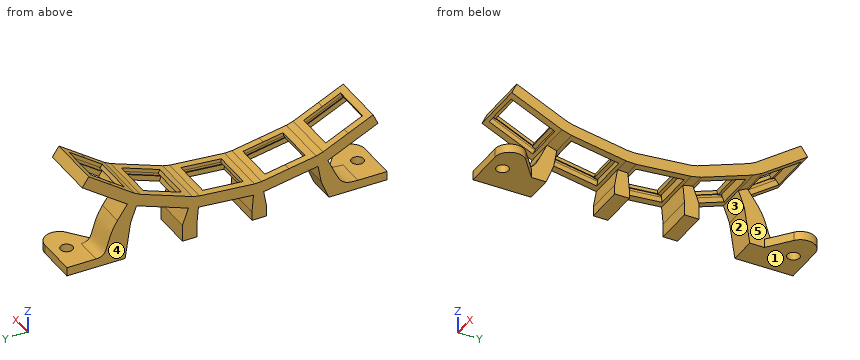
from build123d import *

# Parameters (mm, degrees)
PAD012_DEPTH      = 9.5
POCKET006_DEPTH   = 7
POCKET007_DEPTH   = 7.3
PAD013_DEPTH      = 4.1
PAD013_DEPTH_BACK = 9.5
PAD014_DEPTH      = 9.5
SKETCH025_R       = 2.1
PAD015_DEPTH      = 3


with BuildPart() as part:
    # Sketch020 → Pad012 (new body, symmetric)
    with BuildSketch(Plane.YZ):
        Polygon((-50.2140974459, 25.1635701277), (-41.604173469, 21.1486966411), (-32.9942494922, 17.1338231546), (-30.6406576873, 16.391738509), (-21.2849840337, 14.7420808212), (-11.9293103801, 13.0924231333), (-9.4638496319, 12.9847787924), (0, 13.8127583485), (9.4638496319, 14.6407379046), (11.8731622478, 15.1748696522), (20.8002421453, 18.4240610138), (29.7273220428, 21.6732523754), (31.9162958532, 22.8127600156), (39.698240274, 28.2617361609), (47.4801846947, 33.7107123063), (49.7744904401, 30.4341041291), (34.2106015986, 19.5361518385), (31.0954026161, 17.9144818922), (13.2412428211, 11.416099169), (9.8124726029, 10.6559591122), (-9.1152266609, 9), (-12.6239030908, 9.1531921213), (-31.335250398, 12.452507497), (-34.6847225392, 13.5085920065), (-51.9045704929, 21.5383389795), align=None)
    extrude(amount=PAD012_DEPTH, both=True)

    # Sketch021 → Pocket006 (cut, symmetric)
    with BuildSketch(Plane.YZ):
        Polygon((-47.9483279783, 24.1070244733), (-41.604173469, 21.1486966411), (-35.2600189598, 18.190368809), (-35.8516845262, 16.9215379071), (-34.6734844031, 16.3721341668), (-35.7722918836, 14.0157339205), (-43.294646516, 17.523465493), (-50.8170011484, 21.0311970654), (-49.7181936679, 23.3875973117), (-48.5399935447, 22.8381935715), align=None)
        Polygon((-30.1534810944, 12.2441296838), (-29.7019958324, 14.8046298416), (-28.4217457535, 14.5788872106), (-28.1786383048, 15.9576180648), (-21.2849840337, 14.7420808212), (-14.3913297626, 13.5265435775), (-14.6344372114, 12.1478127233), (-13.3541871324, 11.9220700923), (-13.8056723944, 9.3615699345), (-21.9795767444, 10.8028498091), align=None)
        Polygon((-8.1463979543, 11.6946931063), (-6.8513448468, 11.8079955719), (-6.9733628866, 13.2026681492), (0, 13.8127583485), (6.9733628866, 14.4228485477), (7.0953809265, 13.0281759704), (8.390434034, 13.1414784359), (8.6170389652, 10.5513722209), (0.348622971, 9.8279795561), (-7.9197930232, 9.1045868913), align=None)
        Polygon((14.2223937998, 16.0299200105), (20.8002421453, 18.4240610138), (27.3780904908, 20.818202017), (27.8569186914, 19.5026323479), (29.0785190985, 19.9472585343), (29.9677714711, 17.5040577202), (22.1683227186, 14.6652905306), (14.3688739661, 11.826523341), (13.4796215934, 14.2697241551), (14.7012220004, 14.7143503414), align=None)
        Polygon((33.7022853173, 22.3542388772), (34.7671829748, 23.0998882445), (33.964175964, 24.2467011065), (39.698240274, 28.2617361609), (45.432304584, 32.2767712154), (46.2353115949, 31.1299583534), (47.3002092525, 31.8756077207), (48.791507987, 29.7458124055), (41.9925460194, 24.9851279838), (35.1935840518, 20.2244435621), align=None)
    extrude(amount=POCKET006_DEPTH, both=True, mode=Mode.SUBTRACT)

    # Sketch022 → Pocket007 (cut, symmetric)
    with BuildSketch(Plane.YZ):
        Polygon((-48.4554698924, 23.0194551289), (-35.7671608739, 17.1027994645), (-35.8516845262, 16.9215379071), (-34.6734844031, 16.3721341668), (-35.0115790125, 15.6470879372), (-50.0562882773, 22.6625510822), (-49.7181936678, 23.3875973117), (-48.5399935447, 22.8381935715), align=None)
        Polygon((-28.387016118, 14.7758487612), (-14.5997075758, 12.3447742739), (-14.6344372114, 12.1478127233), (-13.3541871325, 11.9220700923), (-13.4931056746, 11.1342238899), (-29.8409143746, 14.0167836392), (-29.7019958324, 14.8046298416), (-28.4217457535, 14.5788872107), align=None)
        Polygon((-6.8687759954, 12.0072345116), (7.077949778, 13.2274149099), (7.0953809265, 13.0281759703), (8.390434034, 13.1414784359), (8.4601586282, 12.3445226773), (-8.0766733601, 10.8977373481), (-8.1463979543, 11.6946931063), (-6.8513448468, 11.8079955719), align=None)
        Polygon((14.6328179716, 14.9022888661), (27.788514663, 19.6905708716), (27.8569186915, 19.5026323479), (29.0785190985, 19.9472585342), (29.3521352133, 19.1955044372), (13.7532377079, 13.5179700589), (13.4796215934, 14.269724155), (14.7012220005, 14.7143503413), align=None)
        Polygon((34.6524676876, 23.2637186533), (46.1205963076, 31.2937887623), (46.2353115949, 31.1299583534), (47.3002092525, 31.8756077206), (47.7590704015, 31.2202860852), (34.1611464664, 21.6989172418), (33.7022853173, 22.3542388772), (34.7671829749, 23.0998882444), align=None)
    extrude(amount=POCKET007_DEPTH, both=True, mode=Mode.SUBTRACT)

    # Sketch023 → Pad013 (join, two sides)
    with BuildSketch(Plane.YZ) as pad013_sk:
        Polygon((-11.9293103801, 13.0924231333), (-9.4638496319, 12.9847787924), (-9.1152266609, 9), (-8.5922922044, 3.0228318114), (-8.5922922044, 0), (-13.6657921568, 0), (-13.6657921568, 3.2443456032), (-12.6239030908, 9.1531921213), align=None)
        Polygon((9.8124726029, 10.6559591122), (9.4638496319, 14.6407379046), (11.8731622478, 15.1748696522), (13.2412428211, 11.416099169), (15.2933636811, 5.7779434443), (15.2933636811, 0), (10.3354070593, 0), (10.3354070593, 4.6787909237), align=None)
    extrude(amount=PAD013_DEPTH)
    extrude(pad013_sk.sketch, amount=-PAD013_DEPTH_BACK)

    # Sketch024 → Pad014 (join)
    with BuildSketch(Plane.YZ):
        with BuildLine():
            Line((-45, 0), (-35, 0))
            Line((-35, 0), (-32.377139464, 6.5436609789))
            Line((-32.377139464, 6.5436609789), (-31.335250398, 12.452507497))
            Line((-31.335250398, 12.452507497), (-30.6406576873, 16.391738509))
            Line((-30.6406576873, 16.391738509), (-32.9942494922, 17.1338231546))
            Line((-32.9942494922, 17.1338231546), (-34.6847225392, 13.5085920065))
            Line((-34.6847225392, 13.5085920065), (-37.2204321096, 8.0707452842))
            add(Edge.make_bspline(
                [(-37.2204321096, 8.0707452842), (-39.0096732627, 4.233705249), (-40, 3), (-45, 3)],
                knots=[0, 0, 0, 0, 1, 1, 1, 1], degree=3))
            Line((-45, 3), (-45, 0))
        make_face()
        with BuildLine():
            Line((45, 3), (45, 0))
            Line((45, 0), (35, 0))
            Line((35, 0), (33.147523476, 12.2763261675))
            Line((33.147523476, 12.2763261675), (31.0954026161, 17.9144818922))
            Line((31.0954026161, 17.9144818922), (29.7273220428, 21.6732523754))
            Line((29.7273220428, 21.6732523754), (31.9162958532, 22.8127600156))
            Line((31.9162958532, 22.8127600156), (34.2106015986, 19.5361518385))
            Line((34.2106015986, 19.5361518385), (37.6520602167, 14.6212395727))
            add(Edge.make_bspline(
                [(37.6520602167, 14.6212395727), (42.2621193459, 8.0373928164), (40, 3), (45, 3)],
                knots=[0, 0, 0, 0, 1, 1, 1, 1], degree=3))
        make_face()
    extrude(amount=-PAD014_DEPTH)

    # Sketch025 → Pad015 (join)
    with BuildSketch(Plane.XY):
        with BuildLine():
            Line((0, 45), (-9.5, 45))
            Line((-9.5, 45), (-9.5, 55))
            Line((-9.5, 55), (4.5, 55))
            ThreePointArc((7.6224992299, 46.0948753465), (9.218348401, 51.6544450327), (4.5, 55))
            Line((7.6224992299, 46.0948753465), (0, 40))
            Line((0, 45), (0, 40))
        make_face()
        with Locations((0, 50)):
            Circle(SKETCH025_R, mode=Mode.SUBTRACT)
        with BuildLine():
            Line((0, -45), (-9.5, -45))
            Line((-9.5, -45), (-9.5, -55))
            Line((-9.5, -55), (4.5, -55))
            ThreePointArc((4.5, -55), (9.218348401, -51.6544450327), (7.6224992299, -46.0948753465))
            Line((7.6224992299, -46.0948753465), (0, -40))
            Line((0, -40), (0, -45))
        make_face()
        with Locations((0, -50)):
            Circle(SKETCH025_R, mode=Mode.SUBTRACT)
    extrude(amount=PAD015_DEPTH)


with BuildPart() as part_1:
    # Body003 placement: moved
    add(part.part.moved(Location((70, 5, 0))))


solid = part_1.part
Design review of the part built by this model. Coordinates are the model's own, in mm. Face numbers are marked on the shaded views. A direction names the side the tool comes from. Give positions to 0.01 mm unless a question says otherwise; leave off trailing zeros. Write each loop counter-clockwise with the first axis right and the second up, starting at its lowest first coordinate (ties: lowest second). Pieces come first, ordered by that corner, then holes. Notation, with made-up numbers: M -1,43.25 L 22,43.25 A30 ccw 22,76.25 Z; hole C -17,33 d3. An arc over 180 degrees is marked long. Answer as a JSON object with one key per item and string values. Group by question number.
1) For line 1 along X through (y, z) = (-32, 15.5); line 2 along X through (y, z) = (-5.5, 5); line 3 along Y through (x, z) = (66.5, 23), list the stretches that pass through material, from the lowest coordinate up.
2) We need section B-B (x = 64.5). Count the separate pieces of the cut face and the enclosed holes in it, and give its area (3 significant figures).
3) Mouldability with a two-part tool opening along X and no side actions: class the marked faces 3, 4 and 5 as released by +X, released by -X, zero draft, split by the parting line, or undercut.
4) We need section A-A (y = 24). Give the boundary of the cut face in (x, z), and give its area (3 significant figures).
5) Tool access review of the marked faces 1 and 2: name each direction out of +Z, -Z, +X, -X, +Y, -Y from which nothing blocks a thin tool from reaching the whole face with its end or side.
6) Clearance check with flat-ended pins moving along their axes: pin 1 Ø1.5 at (x, z) = (73, 15) entering from +Y; pin 2 Ø10 at (x, y) = (63, 29) entering from +Z; pin 3 Ø2 at (x, z) = (68, 4.5) entering from +Y; pin 4 Ø8 at (y, z) = (49, 26) entering from -X. State where each tip first meets the part, or that it passes through.
Answer key:
{
 "1": {"line 1": "x = 60.5 to 63, 77 to 79.5", "line 2": "x = 60.5 to 74.1", "line 3": "y = -46.22 to -44.9, -43.89 to -43.46, 37.18 to 39.62"},
 "2": {"separate pieces": "6", "enclosed holes": "0", "area": "480 mm²"},
 "3": {"face 3": "zero draft", "face 4": "released by -X", "face 5": "released by +X"},
 "4": {"outline": "M 60.5,13.51 L 63,13.51 L 63,15.43 L 62.7,15.43 L 62.7,16.49 L 63,16.49 L 63,17.77 L 60.5,17.77 Z; M 77,13.51 L 79.5,13.51 L 79.5,17.77 L 77,17.77 L 77,16.49 L 77.3,16.49 L 77.3,15.43 L 77,15.43 Z", "area": "20.6 mm²"},
 "5": {"face 1": "-Z, +X, -X, +Y, -Y", "face 2": "-Z, +X, -X"},
 "6": {"pin 1": "stops at y = 19.7", "pin 2": "stops at z = 21.41", "pin 3": "stops at y = 47.87", "pin 4": "stops at x = 60.5"}
}
